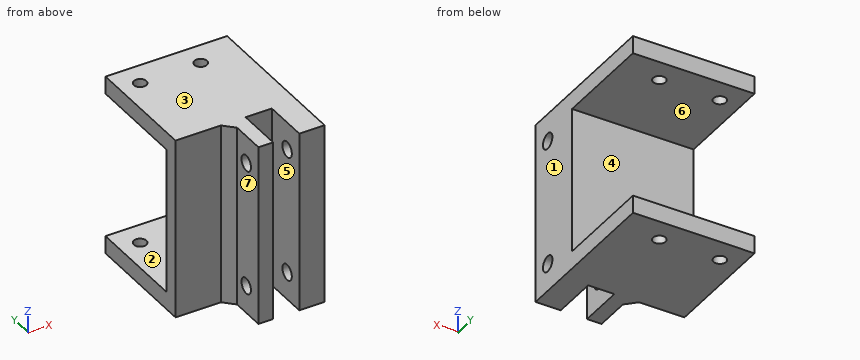
Autodesk Inventor part; units mm, degrees
ref_plane "YZ Plane" through (0, 0, 0) normal (1, 0, 0) x (0, 1, 0)
ref_plane "XZ Plane" through (0, 0, 0) normal (0, 1, 0) x (-1, 0, 0)
ref_plane "XY Plane" through (0, 0, 0) normal (0, 0, 1) x (1, 0, 0)
sketch "Sketch1" plane through (0, 0, 0) normal (0, 1, 0) x (-1, 0, 0)
  line L0 (0, 14.5) -> (22, 14.5)
  line L1 (22, 14.5) -> (22, -14.5)
  line L2 (22, -14.5) -> (0, -14.5)
  line L3 (0, -14.5) -> (0, 14.5)
  circle A0 centre (5, 8) radius 1.25
  circle A1 centre (5, -8) radius 1.25
  circle A2 centre (17, 8) radius 1.25
  circle A3 centre (17, -8) radius 1.25
  line L4 (0, 14.5) -> (22, 14.5)
  line L5 (22, 14.5) -> (22, 17.5)
  line L6 (22, 17.5) -> (0, 17.5)
  line L7 (0, 17.5) -> (0, 14.5)
  line L8 (0, -14.5) -> (22, -14.5)
  line L9 (22, -14.5) -> (22, -17.5)
  line L10 (22, -17.5) -> (0, -17.5)
  line L11 (0, -17.5) -> (0, -14.5)
  point P0 (0, 0)
  dimension "d0" = 29
  dimension "d1" = 14.5
  dimension "d3" = 2.5
  dimension "d4" = 2.5
  dimension "d5" = 16
  dimension "d6" = 8
  dimension "d7" = 5
  dimension "d8" = 5
  dimension "d9" = 2.5
  dimension "d10" = 2.5
  dimension "d11" = 12
  dimension "d12" = 12
  dimension "d13" = 5
  dimension "d24" = 3
  dimension "d25" = 3
extrude "Extrusion1" add sketch "Sketch1" along normal blind 3 contours L7 L6 L5 L0 | L0 L1 L2 L3 | L2 L9 L10 L11 | A0 | A1 | A2 | A3
sketch "Sketch2" plane through (0, 0, 0) normal (0, -1, 0) x (1, 0, 0)
  line L0 (-3, 17.5) -> (0, 17.5)
  line L1 (0, 17.5) -> (0, -17.5)
  line L2 (0, -17.5) -> (-3, -17.5)
  line L3 (-3, -17.5) -> (-3, 17.5)
  line L4 (-22, 17.5) -> (0, 17.5)
  line L5 (0, -17.5) -> (-22, -17.5)
  line L6 (-22, 17.5) -> (0, 17.5)
  line L7 (0, -17.5) -> (-22, -17.5)
  line L8 (-8, 17.5) -> (-11, 17.5)
  line L9 (-11, 17.5) -> (-11, -17.5)
  line L10 (-11, -17.5) -> (-8, -17.5)
  line L11 (-8, -17.5) -> (-8, 17.5)
  line L12 (0, 17.5) -> (0, -17.5)
  point P0 (0, 0)
  point P1 (-8, -17.5)
  dimension "d17" = 3
  dimension "d40" = 3
  dimension "d41" = 5
  dimension "d50" = 0
extrude "Extrusion2" add sketch "Sketch2" along normal blind 9 contours L0 L1 L2 L3 | L11 L5 L9 L4
sketch "Sketch5" plane through (0, 3, 0) normal (0, 1, 0) x (1, 0, 0)
  line L0 (-22, -17.5) -> (0, -17.5)
  line L1 (-22, -17.5) -> (0, -17.5)
  line L2 (0, -17.5) -> (0, -14.5)
  line L3 (0, -14.5) -> (-22, -14.5)
  line L4 (-22, -14.5) -> (-22, -17.5)
  line L5 (-22, 17.5) -> (0, 17.5)
  line L6 (0, 17.5) -> (0, 14.5)
  line L7 (0, 14.5) -> (-22, 14.5)
  line L8 (-22, 14.5) -> (-22, 17.5)
  line L9 (0, 17.5) -> (-22, 17.5)
  line L10 (0, -17.5) -> (0, 17.5)
  point P0 (0, 0)
  dimension "d26" = 3
  dimension "d27" = 3
extrude "Extrusion4" add sketch "Sketch5" along normal blind 20
sketch "Sketch6" plane through (0, 0, 17.5) normal (0, 0, 1) x (1, 0, 0)
  circle A0 centre (-18, 18.25) radius 1.25
  line L0 (-22, 0) -> (0, 0) construction
  circle A1 centre (-6, 18.25) radius 1.25
  line L1 (-22, 0) -> (-22, 23)
  line L2 (0, 0) -> (0, 23)
  line L3 (-22, 3) -> (0, 3)
  line L4 (0, 3) -> (-22, 3)
  dimension "d34" = 2.5
  dimension "d53" = 2.5
  dimension "d54" = 4
  dimension "d55" = 6
  dimension "d56" = 15.25
  dimension "d57" = 15.25
extrude "Extrusion5" cut sketch "Sketch6" against normal blind 50
sketch "Sketch8" plane through (0, -9, 17.5) normal (1, 0, 0) x (0, 0, -1)
  circle A0 centre (5, 4) radius 1.55
  circle A1 centre (30, 4) radius 1.55
  line L0 (35, 0) -> (0, 0)
  line L1 (35, 0) -> (0, 0)
  line L2 (35, 0) -> (35, 32)
  line L3 (0, 0) -> (0, 32)
  point P0 (17.5, 9)
  dimension "d42" = 3.1
  dimension "d43" = 3.1
  dimension "d46" = 4
  dimension "d47" = 4
  dimension "d65" = 5
  dimension "d66" = 5
extrude "Extrusion6" cut sketch "Sketch8" against normal blind 100
thicken "Thicken1" operation add thickness 0.1 both sides no extend neighbours yes toward (1, 0, 0) faces at (-3, -1.1836, -3.9835)
thicken "Thicken2" operation add thickness 0.1 both sides no extend neighbours yes toward (-1, 0, 0) faces at (-8, -1.1836, -3.9835)
chamfer "Chamfer1" distance 2 angle 45 1 edges at (-11, 0, 0)
thicken "Thicken3" operation add thickness 2.1 both sides no extend neighbours yes toward (1, 0, 0) faces at (0, 0.6759, -3.7799)
thicken "Thicken4" operation add thickness 0.5 both sides no extend neighbours yes toward (0, 0, 1) faces at (-12.3333, 11.4808, 17.5)
thicken "Thicken5" operation add thickness 0.5 both sides no extend neighbours yes toward (0, 0, -1) faces at (-12.3333, 11.4808, -17.5)
properties part number "Bar_motor_mount"
Here's how the part is built. I have some questions about the finished solid (model axes, mm). Face numbers are marked on the shaded views. A direction names the side the tool comes from. Coordinates: 2 decimals unless noted, no trailing zeros. Order: outer loops, then holes, each group sorted by start corner. A loop starts at its lowest first (then second) coordinate and runs counter-clockwise, first axis right, second up. Notation, with made-up numbers: (34.5, -35.5) - (48.5, -35.5) arc R15 cw to (48.5, -6.5) - close; hole circle Ø3 at (-6.75, 23.5). An arc over 180 degrees is marked (long way). One line per question, with ' | ' between items.
(1) Will these pins go through, and if not, where does the flat tip stop? pin 1 (4.5 mm diameter, centred on x = -18.5, z = -1.5, fed in from -Y); pin 2 (4 mm diameter, centred on y = -5, z = -12.5, fed in from -X); pin 3 (3 mm diameter, centred on y = -5, z = 12.5, fed in from -X).
Report:
pin 1: stops at y = 0 | pin 2: stops at x = -11 | pin 3: passes through
(2) Suppose I cut it at B-B on y = 7.5. List the corners of the cut face in (x, z) for me.
Report:
outline: (-22, -18) - (2.1, -18) - (2.1, -14.5) - (-22, -14.5) - close; (-22, 14.5) - (2.1, 14.5) - (2.1, 18) - (-22, 18) - close
(3) If I drill on L1, parallel to Y at x = -8.85, z = 12.5; L2, parallel to X at y = -2, z = -4; L3, parallel to Z at x = -6.75, y = 5, over which ranges is the centre line in solid material (lowest first)?
Report:
L1: y = -9 to -6.55, -3.45 to 3 | L2: x = -11 to -8.1, -2.9 to 2.1 | L3: z = -18 to -14.5, 14.5 to 18
(4) Suppose I cut it at A-A on x = -18. List the corners of the cut face in (y, z) for me, and give its area (4 significant figures).
Report:
outline: (0, -18) - (17, -18) - (17, -14.5) - (3, -14.5) - (3, 14.5) - (17, 14.5) - (17, 18) - (0, 18) - close; (19.5, -18) - (23, -18) - (23, -14.5) - (19.5, -14.5) - close; (19.5, 14.5) - (23, 14.5) - (23, 18) - (19.5, 18) - close | area: 230.5 mm2
(5) Suppose I cut it at D-D on y = 18.25. List the corners of the cut face in (x, z) for me.
Report:
outline: (-22, -18) - (-19.25, -18) - (-19.25, -14.5) - (-22, -14.5) - close; (-22, 14.5) - (-19.25, 14.5) - (-19.25, 18) - (-22, 18) - close; (-16.75, -18) - (-7.25, -18) - (-7.25, -14.5) - (-16.75, -14.5) - close; (-16.75, 14.5) - (-7.25, 14.5) - (-7.25, 18) - (-16.75, 18) - close; (-4.75, -18) - (2.1, -18) - (2.1, -14.5) - (-4.75, -14.5) - close; (-4.75, 14.5) - (2.1, 14.5) - (2.1, 18) - (-4.75, 18) - close
(6) For the marked faces 5, 6 and 7, which set-ups out of +Z, -Z, +X, -X, +Y, -Y let a thin tool reach every point of the face, with its end or its side?
Report:
face 5: +Z, -Z, -Y | face 6: +X, -X, +Y | face 7: +Z, -Z, -X, -Y
(7) If we mould it in two halves opening along Z, with no side actions, what happens to the marked faces 1, 2, 3 and 4? For each: pulls with the +Z half, pulls with the -Z half, needs draft (parallel to the pull), parting line crosses it, or undercut.
Report:
face 1: needs draft | face 2: undercut | face 3: pulls with the +Z half | face 4: undercut
(8) Suppose I cut it at C-C on z = -12.5. List the corners of the cut face in (x, y) for me, and give its area (3 significant figures).
Report:
outline: (-22, 0) - (-13, 0) - (-11, -2) - (-11, -3.45) - (-8.1, -3.45) - (-8.1, 0) - (-2.9, 0) - (-2.9, -3.45) - (2.1, -3.45) - (2.1, 3) - (-22, 3) - close; (-11, -9) - (-8.1, -9) - (-8.1, -6.55) - (-11, -6.55) - close; (-2.9, -9) - (2.1, -9) - (2.1, -6.55) - (-2.9, -6.55) - close | area: 121 mm2
